```python
from build123d import *

# Parameters (mm, degrees)
SKETCH1_R           = 12.7
BOSS_EXTRUDE1_DEPTH = 0.6985
SKETCH2_R           = 12.7
BOSS_EXTRUDE2_DEPTH = 6.35
BOSS_EXTRUDE2_TAPER = 45
SKETCH3_R           = 4.7625
CUT_EXTRUDE1_DEPTH  = 20.294075706


with BuildPart() as part:
    # Sketch1 → Boss-Extrude1 (new body)
    with BuildSketch(Plane(origin=(0, 0, 0), x_dir=(1, 0, 0), z_dir=(0, 1, 0))):
        with Locations(Location((0, 0, 0), (0, 0, 270))):
            Circle(SKETCH1_R)
    extrude(amount=BOSS_EXTRUDE1_DEPTH)

    # Sketch2 → Boss-Extrude2 (add)
    with BuildSketch(Plane(origin=(0, 0.6985, 0), x_dir=(1, 0, 0), z_dir=(0, 1, 0))):
        with Locations(Location((0, 0, 0), (0, 0, 270))):
            Circle(SKETCH2_R)
    extrude(amount=BOSS_EXTRUDE2_DEPTH, taper=BOSS_EXTRUDE2_TAPER)

    # Sketch3 → Cut-Extrude1 (cut, through all)
    with BuildSketch(Plane(origin=(0, 7.0485, 0), x_dir=(1, 0, 0), z_dir=(0, 1, 0))):
        with Locations(Location((0, 0, 0), (0, 0, 270))):
            Circle(SKETCH3_R)
    extrude(amount=-CUT_EXTRUDE1_DEPTH, mode=Mode.SUBTRACT)


solid = part.part
```
Geometry check sheet. Reference: the model listing, model coordinates, mm. Coordinates: 2 decimals unless noted, no trailing zeros. Loops run counter-clockwise (first coordinate to the right, second up) from the corner with the lowest first, then second, coordinate; pieces in that order, holes last.
Item 1: Release check for a two-part mould opening along Z. For faces 1 (the face through (2, 6.74, 6.35)), 2 (the face through (5, 7.048, 1)), 3 (the face through (-2.9, 3.57, -3.78)) record: released by +Z, released by -Z, zero draft, split by the parting line, or undercut.
Item 2: Sectioned sample at C-C, the plane y = 2. Record the boundary of the cut face in (x, z) (1 decimal).
Item 3: Thickness scan on line 1 (Z direction, x = -2.5, y = 4.75); line 2 (X direction, y = 4.5, z = 0); line 3 (Z direction, x = -1, y = 5.5). Record the ranges inside material, lowest first.
Item 4: Go/stop test with flat-tipped pins: pin 1 Ø2 at (x, z) = (5.5, -7.5) entering from +Y; pin 2 Ø1.5 at (y, z) = (6, 3) entering from +X; pin 3 Ø2 at (y, z) = (6, 1.5) entering from -X. Record where each tip stops, or that it passes through.
Item 5: Sectioned sample at B-B, the plane y = 6.5. Record the boundary of the cut face in (x, z) (1 decimal).
Item 6: Sectioned sample at A-A, the plane z = 0. Record the boundary of the cut face in (x, y).
Check result:
1. face 1: split by the parting line
1. face 2: zero draft
1. face 3: undercut
2. outline: circle Ø22.8 at (0, 0); hole circle Ø9.5 at (0, 0)
3. line 1: z = -8.28 to -4.05, 4.05 to 8.28
3. line 2: x = -8.9 to -4.76, 4.76 to 8.9
3. line 3: z = -7.83 to -4.66, 4.66 to 7.83
4. pin 1: stops at y = 5.1
4. pin 2: stops at x = 7.62
4. pin 3: stops at x = -8.28
5. outline: circle Ø13.8 at (0, 0); hole circle Ø9.5 at (0, 0)
6. outline: (-12.7, 0) - (-4.76, 0) - (-4.76, 7.05) - (-6.35, 7.05) - (-12.7, 0.7) - close; (4.76, 0) - (12.7, 0) - (12.7, 0.7) - (6.35, 7.05) - (4.76, 7.05) - close
